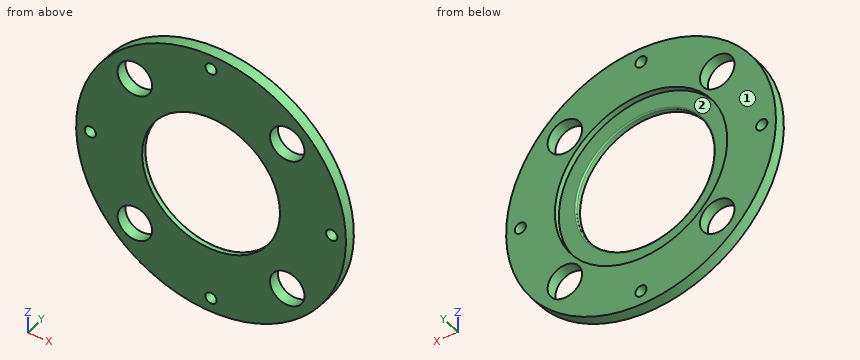
```python
from build123d import *

# Parameters (mm, degrees)
SKETCH1_R           = 46.95
SKETCH1_R_2         = 1.95
SKETCH1_R_3         = 30
BOSS_EXTRUDE1_DEPTH = 2
SKETCH2_R           = 30
SKETCH2_R_2         = 24
BOSS_EXTRUDE2_DEPTH = 2
CUT_EXTRUDE1_START  = -33
SKETCH3_R           = 1.95
SKETCH3_R_2         = 6
CUT_EXTRUDE1_DEPTH  = 33
FILLET1_R           = 0.5


with BuildPart() as part:
    # Sketch1 → Boss-Extrude1 (new, symmetric)
    with BuildSketch(Plane(origin=(0, 0, 0), x_dir=(1, 0, 0), z_dir=(0, 1, 0))):
        with Locations(Location((0, 0, 0), (0, 0, 270))):
            Circle(SKETCH1_R)
        with Locations(Location((0, 42, 0), (0, 0, 270))):
            Circle(SKETCH1_R_2, mode=Mode.SUBTRACT)
        with Locations(Location((42, 0, 0), (0, 0, 270))):
            Circle(SKETCH1_R_2, mode=Mode.SUBTRACT)
        with Locations(Location((0, -42, 0), (0, 0, 270))):
            Circle(SKETCH1_R_2, mode=Mode.SUBTRACT)
        with Locations(Location((-42, 0, 0), (0, 0, 270))):
            Circle(SKETCH1_R_2, mode=Mode.SUBTRACT)
        with Locations(Location((0, 0, 0), (0, 0, 270))):
            Circle(SKETCH1_R_3, mode=Mode.SUBTRACT)
    extrude(amount=BOSS_EXTRUDE1_DEPTH, both=True)

    # Sketch2 → Boss-Extrude2 (add)
    with BuildSketch(Plane.XZ.offset(2)):
        with Locations(Location((0, 0, 0), (0, 0, 90))):
            Circle(SKETCH2_R)
        with Locations(Location((0, 0, 0), (0, 0, 270))):
            Circle(SKETCH2_R_2, mode=Mode.SUBTRACT)
    extrude(amount=-BOSS_EXTRUDE2_DEPTH)

    # Sketch3 → Cut-Extrude1 (cut)
    with BuildSketch(Plane(origin=(0, 2, 0), x_dir=(1, 0, 0), z_dir=(0, 1, 0)).offset(CUT_EXTRUDE1_START)):
        with Locations(Location((-42, 0, 0), (0, 0, 270))):
            Circle(SKETCH3_R)
        with Locations(Location((-26.516504294, 26.516504294, 0), (0, 0, 270))):
            Circle(SKETCH3_R_2)
        with Locations(Location((26.516504294, 26.516504294, 0), (0, 0, 270))):
            Circle(SKETCH3_R_2)
        with Locations(Location((26.516504294, -26.516504294, 0), (0, 0, 270))):
            Circle(SKETCH3_R_2)
        with Locations(Location((-26.516504294, -26.516504294, 0), (0, 0, 270))):
            Circle(SKETCH3_R_2)
    extrude(amount=CUT_EXTRUDE1_DEPTH, mode=Mode.SUBTRACT)

    # Fillet1
    fillet1_edges = [part.edges().sort_by_distance(p)[0] for p in [
        (0, 0, 24),
    ]]
    fillet(fillet1_edges, radius=FILLET1_R)


solid = part.part
```
Input: part model. Units: mm. Frame: model coordinates. Face numbers are marked on the shaded views. Give positions to 0.01 mm unless a question says otherwise; leave off trailing zeros. Order: outer loops, then holes, each group sorted by start corner. A loop starts at its lowest first (then second) coordinate and runs counter-clockwise, first axis right, second up.
1. Section C-C on x = 42. Return the cut outline in (y, z), and give its area (3 significant figures).
Derived:
outline: (-2, -20.98) - (2, -20.98) - (2, -1.95) - (-2, -1.95) - close; (-2, 1.95) - (2, 1.95) - (2, 20.98) - (-2, 20.98) - close
area: 152 mm2
2. Material intervals for L1, parallel to X at y = 1.05, z = 0; L2, parallel to X at y = -0.1, z = -28.5, sorted ascending.
Derived:
L1: x = -46.95 to -43.95, -40.05 to -30, 30 to 40.05, 43.95 to 46.95
L2: x = -37.31 to -32.18, -20.85 to 20.85, 32.18 to 37.31
3. Pin query (flat end, axial travel): pin 1 (4.5 mm diameter, centred on x = 42, z = 0, fed in from -Y). Return the tip coordinate at first contact, or that it passes through.
Derived:
pin 1: stops at y = -2
4. Section D-D on y = 1.25. Give the number of separate pieces and of enclosed holes in the cut face, and give its area (3 significant figures).
Derived:
separate pieces: 1
enclosed holes: 9
area: 3,600 mm2
5. Mould query, pull axis X, two halves, no side actions, for the marked faces 1 and 2. Classes: released by +X, released by -X, zero draft, split by the parting line, or undercut.
Derived:
face 1: zero draft
face 2: undercut
6. Section A-A on z = 0. Return the cut outline in (x, y), and give its area (3 significant figures).
Derived:
outline: (-46.95, -2) - (-43.95, -2) - (-43.95, 2) - (-46.95, 2) - close; (-40.05, -2) - (-24, -2) - (-24, -0.5) arc R0.5 ccw to (-24.5, 0) - (-30, 0) - (-30, 2) - (-40.05, 2) - close; (24, -2) - (40.05, -2) - (40.05, 2) - (30, 2) - (30, 0) - (24.5, 0) arc R0.5 ccw to (24, -0.5) - close; (43.95, -2) - (46.95, -2) - (46.95, 2) - (43.95, 2) - close
area: 128 mm2
7. Section B-B on x = 0. Return the cut outline in (y, z), and give its area (3 significant figures).
Derived:
outline: (-2, -46.95) - (2, -46.95) - (2, -43.95) - (-2, -43.95) - close; (-2, -40.05) - (2, -40.05) - (2, -30) - (0, -30) - (0, -24.5) arc R0.5 ccw to (-0.5, -24) - (-2, -24) - close; (-2, 24) - (-0.5, 24) arc R0.5 ccw to (0, 24.5) - (0, 30) - (2, 30) - (2, 40.05) - (-2, 40.05) - close; (-2, 43.95) - (2, 43.95) - (2, 46.95) - (-2, 46.95) - close
area: 128 mm2
